from build123d import *
from OCP.BRepFilletAPI import BRepFilletAPI_MakeChamfer

# Parameters (mm, degrees)
SKETCH1_W           = 53
SKETCH1_H           = 5
SKETCH1_H_2         = 70
SKETCH1_R           = 1.5
BOSS_EXTRUDE1_DEPTH = 5
SKETCH2_R           = 1.5
CUT_EXTRUDE1_DEPTH  = 10
SKETCH3_R           = 3.5
CUT_EXTRUDE2_DEPTH  = 3
SKETCH2_3_W         = 2.25
SKETCH2_3_H         = 15
BOSS_EXTRUDE2_DEPTH = 6
CUT_EXTRUDE3_DEPTH  = 79.961729873
CHAMFER2_SIZE       = 0.75
CHAMFER2_SIZE_2     = 4.253461365
CHAMFER3_SIZE       = 1.1
CHAMFER3_SIZE_2     = 6.238410002
SKETCH5_W           = 15
SKETCH5_H           = 30
CUT_EXTRUDE4_DEPTH  = 3
FILLET1_R           = 10
CHAMFER4_SIZE       = 5


# Some blends are built 0.0001 mm under size
with BuildPart() as part:
    # Sketch1 → Boss-Extrude1 (new body)
    # profile 1 of 2: a face of its own
    with BuildSketch(Plane(origin=(0, 0, 0), x_dir=(1, 0, 0), z_dir=(0, 1, 0))):
        with Locations((5.35835502, -40.562169312)):
            Rectangle(SKETCH1_W, SKETCH1_H)
    # profile 2 of 2: a face of its own
    with BuildSketch(Plane(origin=(0, 0, 0), x_dir=(1, 0, 0), z_dir=(0, 1, 0))):
        with Locations((5.35835502, -3.062169312)):
            Rectangle(SKETCH1_W, SKETCH1_H_2)
        with Locations(Location((29.35835502, -24.362169312, 0), (0, 0, 270))):
            Circle(SKETCH1_R, mode=Mode.SUBTRACT)
        with Locations(Location((24.85835502, 27.437830688, 0), (0, 0, 270))):
            Circle(SKETCH1_R, mode=Mode.SUBTRACT)
        with Locations(Location((-3.14164498, 27.437830688, 0), (0, 0, 270))):
            Circle(SKETCH1_R, mode=Mode.SUBTRACT)
        with Locations(Location((-18.64164498, -23.062169312, 0), (0, 0, 270))):
            Circle(SKETCH1_R, mode=Mode.SUBTRACT)
    extrude(amount=BOSS_EXTRUDE1_DEPTH)

    # Sketch2 → Cut-Extrude1 (cut)
    with BuildSketch(Plane.XZ):
        with Locations(Location((5.35835502, 15.062169312, 0), (0, 0, 270))):
            Circle(SKETCH2_R)
    extrude(amount=-CUT_EXTRUDE1_DEPTH, mode=Mode.SUBTRACT)

    # Sketch3 → Cut-Extrude2 (cut)
    with BuildSketch(Plane(origin=(0, 5, 0), x_dir=(1, 0, 0), z_dir=(0, 1, 0))):
        with Locations(Location((5.35835502, -15.062169312, 0), (0, 0, 270))):
            Circle(SKETCH3_R)
    extrude(amount=-CUT_EXTRUDE2_DEPTH, mode=Mode.SUBTRACT)

    # Sketch2<3> → Boss-Extrude2 (add)
    with BuildSketch(Plane.XZ):
        with Locations((3.48335502, -2.437830688)):
            Rectangle(SKETCH2_3_W, SKETCH2_3_H)
        with Locations((7.23335502, -2.437830688)):
            Rectangle(SKETCH2_3_W, SKETCH2_3_H)
        with Locations((7.23335502, 32.562169312)):
            Rectangle(SKETCH2_3_W, SKETCH2_3_H)
        with Locations((3.48335502, 32.562169312)):
            Rectangle(SKETCH2_3_W, SKETCH2_3_H)
    extrude(amount=BOSS_EXTRUDE2_DEPTH)

    # Sketch4 → Cut-Extrude3 (cut, through all)
    with BuildSketch(Plane.XY.offset(40.062169312)):
        Polygon((8.35835502, -4.5), (8.35835502, 0), (7.65835502, 0), (7.65835502, -4), (8.05835502, -4.285714286), (8.05835502, -5.1), (7.15835502, -6), (8.35835502, -6), (8.35835502, -4.8), align=None)
        Polygon((2.65835502, -4.285714286), (3.05835502, -4), (3.05835502, 0), (2.35835502, 0), (2.35835502, -4.5), (2.35835502, -4.8), (2.35835502, -6), (3.55835502, -6), (2.65835502, -5.1), align=None)
    extrude(amount=-CUT_EXTRUDE3_DEPTH, mode=Mode.SUBTRACT)

    # Chamfer2
    chamfer2_edges_1 = [part.edges().sort_by_distance(p)[0] for p in [
        (4.60835502, 0, -2.437830688),
    ]]
    chamfer2_side_1 = [part.faces().sort_by_distance(p)[0] for p in [
        (4.62335502, 0, -2.437830688),
    ]]
    chamfer2_edges_2 = [part.edges().sort_by_distance(p)[0] for p in [
        (6.10835502, 0, -2.437830688),
    ]]
    chamfer2_side_2 = [part.faces().sort_by_distance(p)[0] for p in [
        (6.09335502, 0, -2.437830688),
    ]]
    chamfer2_edges_3 = [part.edges().sort_by_distance(p)[0] for p in [
        (6.10835502, 0, 32.562169312),
    ]]
    chamfer2_side_3 = [part.faces().sort_by_distance(p)[0] for p in [
        (6.09335502, 0, 32.562169312),
    ]]
    chamfer2_edges_4 = [part.edges().sort_by_distance(p)[0] for p in [
        (4.60835502, 0, 32.562169312),
    ]]
    chamfer2_side_4 = [part.faces().sort_by_distance(p)[0] for p in [
        (4.62335502, 0, 32.562169312),
    ]]
    chamfer2 = BRepFilletAPI_MakeChamfer(part.part.solid().wrapped)
    for e in chamfer2_edges_1:
        chamfer2.Add(CHAMFER2_SIZE - 0.0001, CHAMFER2_SIZE_2 - 0.0001, e.wrapped, chamfer2_side_1[0].wrapped)
    for e in chamfer2_edges_2:
        chamfer2.Add(CHAMFER2_SIZE - 0.0001, CHAMFER2_SIZE_2 - 0.0001, e.wrapped, chamfer2_side_2[0].wrapped)
    for e in chamfer2_edges_3:
        chamfer2.Add(CHAMFER2_SIZE - 0.0001, CHAMFER2_SIZE_2 - 0.0001, e.wrapped, chamfer2_side_3[0].wrapped)
    for e in chamfer2_edges_4:
        chamfer2.Add(CHAMFER2_SIZE - 0.0001, CHAMFER2_SIZE_2 - 0.0001, e.wrapped, chamfer2_side_4[0].wrapped)
    add(Compound.cast(chamfer2.Shape()), mode=Mode.REPLACE)  # a hair under: the kernel refuses the full size

    # Chamfer3
    # the kernel refuses this chamfer: 6.238410002, 1.1 mm, written as the material it takes off along each edge
    with BuildSketch(Plane(origin=(20.819105437, -6, 40.062169312), x_dir=(0, -0.210138760767435, -0.977671571246258), z_dir=(-1, 0, 0))) as chamfer3_piece_1_section:
        Polygon((CHAMFER3_SIZE * 0.977671571246, -CHAMFER3_SIZE * 0.210138760767), (-CHAMFER3_SIZE_2 * 0.210138760753, -CHAMFER3_SIZE_2 * 0.97767157118), (0, 0), align=None)
    chamfer3_piece_1 = extrude(amount=33.471500834, mode=Mode.PRIVATE)
    chamfer3_piece_1 = split(chamfer3_piece_1, bisect_by=Plane(origin=(4.08335502, 0, 39.758425896), z_dir=(0, -1, 0)), keep=Keep.TOP, mode=Mode.PRIVATE)
    add(chamfer3_piece_1, mode=Mode.SUBTRACT)
    with BuildSketch(Plane(origin=(-12.652395397, -6, 25.062169312), x_dir=(0, -0.210138760767435, 0.977671571246258), z_dir=(1, 0, 0))) as chamfer3_piece_2_section:
        Polygon((CHAMFER3_SIZE * 0.977671571246, -CHAMFER3_SIZE * 0.210138760767), (-CHAMFER3_SIZE_2 * 0.210138760753, -CHAMFER3_SIZE_2 * 0.97767157118), (0, 0), align=None)
    chamfer3_piece_2 = extrude(amount=33.471500834, mode=Mode.PRIVATE)
    chamfer3_piece_2 = split(chamfer3_piece_2, bisect_by=Plane(origin=(4.08335502, 0, 25.365912729), z_dir=(0, -1, 0)), keep=Keep.TOP, mode=Mode.PRIVATE)
    add(chamfer3_piece_2, mode=Mode.SUBTRACT)
    with BuildSketch(Plane(origin=(23.369105437, -6, 40.062169312), x_dir=(0, -0.210138760767435, -0.977671571246258), z_dir=(-1, 0, 0))) as chamfer3_piece_3_section:
        Polygon((CHAMFER3_SIZE * 0.977671571246, -CHAMFER3_SIZE * 0.210138760767), (-CHAMFER3_SIZE_2 * 0.210138760753, -CHAMFER3_SIZE_2 * 0.97767157118), (0, 0), align=None)
    chamfer3_piece_3 = extrude(amount=33.471500834, mode=Mode.PRIVATE)
    chamfer3_piece_3 = split(chamfer3_piece_3, bisect_by=Plane(origin=(6.63335502, 0, 39.758425896), z_dir=(0, -1, 0)), keep=Keep.TOP, mode=Mode.PRIVATE)
    add(chamfer3_piece_3, mode=Mode.SUBTRACT)
    with BuildSketch(Plane(origin=(-10.102395397, -6, 25.062169312), x_dir=(0, -0.210138760767435, 0.977671571246258), z_dir=(1, 0, 0))) as chamfer3_piece_4_section:
        Polygon((CHAMFER3_SIZE * 0.977671571246, -CHAMFER3_SIZE * 0.210138760767), (-CHAMFER3_SIZE_2 * 0.210138760753, -CHAMFER3_SIZE_2 * 0.97767157118), (0, 0), align=None)
    chamfer3_piece_4 = extrude(amount=33.471500834, mode=Mode.PRIVATE)
    chamfer3_piece_4 = split(chamfer3_piece_4, bisect_by=Plane(origin=(6.63335502, 0, 25.365912729), z_dir=(0, -1, 0)), keep=Keep.TOP, mode=Mode.PRIVATE)
    add(chamfer3_piece_4, mode=Mode.SUBTRACT)
    with BuildSketch(Plane(origin=(23.369105437, -6, 5.062169312), x_dir=(0, -0.21013876076743537, -0.9776715712462578), z_dir=(-1, 0, 0))) as chamfer3_piece_5_section:
        Polygon((CHAMFER3_SIZE * 0.977671571246, -CHAMFER3_SIZE * 0.210138760767), (-CHAMFER3_SIZE_2 * 0.210138760753, -CHAMFER3_SIZE_2 * 0.97767157118), (0, 0), align=None)
    chamfer3_piece_5 = extrude(amount=33.471500834, mode=Mode.PRIVATE)
    chamfer3_piece_5 = split(chamfer3_piece_5, bisect_by=Plane(origin=(6.63335502, 0, 4.758425896), z_dir=(0, -1, 0)), keep=Keep.TOP, mode=Mode.PRIVATE)
    add(chamfer3_piece_5, mode=Mode.SUBTRACT)
    with BuildSketch(Plane(origin=(-10.102395397, -6, -9.937830688), x_dir=(0, -0.21013876076743562, 0.9776715712462578), z_dir=(1, 0, 0))) as chamfer3_piece_6_section:
        Polygon((CHAMFER3_SIZE * 0.977671571246, -CHAMFER3_SIZE * 0.210138760767), (-CHAMFER3_SIZE_2 * 0.210138760753, -CHAMFER3_SIZE_2 * 0.97767157118), (0, 0), align=None)
    chamfer3_piece_6 = extrude(amount=33.471500834, mode=Mode.PRIVATE)
    chamfer3_piece_6 = split(chamfer3_piece_6, bisect_by=Plane(origin=(6.63335502, 0, -9.634087271), z_dir=(0, -1, 0)), keep=Keep.TOP, mode=Mode.PRIVATE)
    add(chamfer3_piece_6, mode=Mode.SUBTRACT)
    with BuildSketch(Plane(origin=(20.819105437, -6, 5.062169312), x_dir=(0, -0.21013876076743546, -0.9776715712462578), z_dir=(-1, 0, 0))) as chamfer3_piece_7_section:
        Polygon((CHAMFER3_SIZE * 0.977671571246, -CHAMFER3_SIZE * 0.210138760767), (-CHAMFER3_SIZE_2 * 0.210138760753, -CHAMFER3_SIZE_2 * 0.97767157118), (0, 0), align=None)
    chamfer3_piece_7 = extrude(amount=33.471500834, mode=Mode.PRIVATE)
    chamfer3_piece_7 = split(chamfer3_piece_7, bisect_by=Plane(origin=(4.08335502, 0, 4.758425896), z_dir=(0, -1, 0)), keep=Keep.TOP, mode=Mode.PRIVATE)
    add(chamfer3_piece_7, mode=Mode.SUBTRACT)
    with BuildSketch(Plane(origin=(-12.652395397, -6, -9.937830688), x_dir=(-1.5437276286848704e-15, -0.21013876076743562, 0.9776715712462578), z_dir=(1, 0, 0))) as chamfer3_piece_8_section:
        Polygon((CHAMFER3_SIZE * 0.977671571246, -CHAMFER3_SIZE * 0.210138760767), (-CHAMFER3_SIZE_2 * 0.210138760753, -CHAMFER3_SIZE_2 * 0.97767157118), (0, 0), align=None)
    chamfer3_piece_8 = extrude(amount=33.471500834, mode=Mode.PRIVATE)
    chamfer3_piece_8 = split(chamfer3_piece_8, bisect_by=Plane(origin=(4.08335502, 0, -9.634087271), z_dir=(0, -1, 0)), keep=Keep.TOP, mode=Mode.PRIVATE)
    add(chamfer3_piece_8, mode=Mode.SUBTRACT)

    # Sketch5 → Cut-Extrude4 (cut)
    with BuildSketch(Plane.XZ):
        with Locations((24.35835502, 5.062169312)):
            Rectangle(SKETCH5_W, SKETCH5_H)
        with Locations((-13.64164498, 5.062169312)):
            Rectangle(SKETCH5_W, SKETCH5_H)
    extrude(amount=-CUT_EXTRUDE4_DEPTH, mode=Mode.SUBTRACT)

    # Fillet1
    # the kernel refuses this fillet: 10 mm, written as the material it adds along each edge
    with BuildSketch(Plane(origin=(31.85835502, 3, -9.937830688), x_dir=(0, -1, 0), z_dir=(-1, 0, 0))) as fillet1_piece_1:
        with BuildLine():
            CenterArc((10, 7.141428429), FILLET1_R, 180, 45.572995999)
            Line((0, 7.141428429), (0, 0))
            Line((0, 0), (3, 0))
        make_face()
    extrude(amount=32.853571071)
    with BuildSketch(Plane(origin=(16.85835502, 3, 20.062169312), x_dir=(0, -1, 0), z_dir=(1, 0, 0))) as fillet1_piece_2:
        with BuildLine():
            CenterArc((10, 7.141428429), FILLET1_R, 180, 45.572995999)
            Line((0, 7.141428429), (0, 0))
            Line((0, 0), (3, 0))
        make_face()
    extrude(amount=15)
    with BuildSketch(Plane(origin=(-6.14164498, 3, 20.062169312), x_dir=(0, -1, 0), z_dir=(-1, 0, 0))) as fillet1_piece_3:
        with BuildLine():
            CenterArc((10, -7.141428429), FILLET1_R, 134.427004001, 45.572995999)
            Line((0, -7.141428429), (0, 0))
            Line((0, 0), (3, 0))
        make_face()
    extrude(amount=15)
    with BuildSketch(Plane(origin=(-21.14164498, 3, -9.937830688), x_dir=(0, -1, 0), z_dir=(1, 0, 0))) as fillet1_piece_4:
        with BuildLine():
            CenterArc((10, -7.141428429), FILLET1_R, 134.427004001, 45.572995999)
            Line((0, -7.141428429), (0, 0))
            Line((0, 0), (3, 0))
        make_face()
    extrude(amount=32.853571071)
    with BuildSketch(Plane(origin=(-6.14164498, 3, -27.791401759), x_dir=(0, -1, 0), z_dir=(0, 0, 1))) as fillet1_piece_5:
        with BuildLine():
            CenterArc((10, -7.141428429), FILLET1_R, 134.427004001, 45.572995999)
            Line((0, -7.141428429), (0, 0))
            Line((0, 0), (3, 0))
        make_face()
    extrude(amount=65.707142143)
    with BuildSketch(Plane(origin=(16.85835502, 3, -9.937830688), x_dir=(0, -1, 0), z_dir=(0, 0, 1))) as fillet1_piece_6:
        with BuildLine():
            CenterArc((10, 7.141428429), FILLET1_R, 180, 45.572995999)
            Line((0, 7.141428429), (0, 0))
            Line((0, 0), (3, 0))
        make_face()
    extrude(amount=47.853571071)

    # Chamfer4
    chamfer4_edges = [part.edges().sort_by_distance(p)[0] for p in [
        (31.85835502, 2.5, 43.062169312),
        (-21.14164498, 2.5, 43.062169312),
        (-21.14164498, 2.5, -31.937830688),
        (31.85835502, 2.5, -31.937830688),
    ]]
    chamfer(chamfer4_edges, length=CHAMFER4_SIZE)


solid = part.part
Can you work these out from the model? Positions are in its coordinate system, mm. A direction names the side the tool comes from. Coordinates: 2 decimals unless noted, no trailing zeros. Order: outer loops, then holes, each group sorted by start corner. A loop starts at its lowest first (then second) coordinate and runs counter-clockwise, first axis right, second up. Notation, with made-up numbers: (-22, 65) -> (29, 65) arc R7 ccw to (29, 69) -> close; hole circle Ø2 at (67, -7). An arc over 180 degrees is marked (long way). Use one line per item in the form item = value.
Q1. I need wall thicknesses on L1, parallel to Y at x = -6, z = 17; L2, parallel to X at y = -4.75, z = 39; L3, parallel to X at y = -1, z = 30.5. Which ranges of each line are inside material? Lowest first, please.
From the geometry:
L1 = 0 to 5
L2 = 2.66 to 4.61, 6.11 to 8.06
L3 = 3.06 to 5.18, 5.53 to 7.66
Q2. Imagine slicing it at A-A, the plane y = -1.5. List the corners of the cut face in (x, z) for me, then the cut area to 3 significant figures.
From the geometry:
outline = (3.06, -9.63) -> (5.09, -9.63) -> (5.09, 4.76) -> (3.06, 4.76) -> close; (3.06, 25.37) -> (5.09, 25.37) -> (5.09, 39.76) -> (3.06, 39.76) -> close; (5.62, -9.63) -> (7.66, -9.63) -> (7.66, 4.76) -> (5.62, 4.76) -> close; (5.62, 25.37) -> (7.66, 25.37) -> (7.66, 39.76) -> (5.62, 39.76) -> close
area = 117 mm²
Q3. Imagine slicing it at C-C, the plane x = 15.5. List the corners of the cut face in (y, z) for me.
From the geometry:
outline = (0, -31.94) -> (5, -31.94) -> (5, 43.06) -> (0, 43.06) -> close
Q4. Which directions (+Z, -Z, +X, -X, +Y, -Y) give clear straight access to the entire face, cutting with the end or side of a thin tool? Please do faces 1 (the face through (7.658, -2, 33)), 2 (the face through (6.108, -5, -3)), 3 (the face through (-15.41, 2.2, -6.72)).
From the geometry:
face_1 = +Z, -Z, +X
face_2 = +Z, -Z, -Y
face_3 = -X, -Y
Q5. Imagine slicing it at D-D, the plane z = 7.5. List the corners of the cut face in (x, y) for me, then the cut area to 3 significant figures.
From the geometry:
outline = (-21.14, 3) -> (-13.28, 3) arc R10 cw to (-6.14, 0) -> (16.86, 0) arc R10 cw to (24, 3) -> (31.86, 3) -> (31.86, 5) -> (-21.14, 5) -> close
area = 188 mm²
Q6. We'd pull the mould along Z, two halves only. Please class faces 4 (the face through (-4.606, 2.465, -27.763)), 5 (the face through (5, 2, 17)), 6 (the face through (-18.607, 2.465, 40.597)), 7 (the face through (-21.142, 4, 5)): released by +Z, released by -Z, zero draft, split by the parting line, or undercut.
From the geometry:
face_4 = undercut
face_5 = undercut
face_6 = released by +Z
face_7 = zero draft
Q7. Will these pins go through, and if not, where does the flat tip stop? P1, Ø4, axis at y = 1.5, z = 10.5, coming from the +X side; P2, Ø4, axis at x = 5.36, z = 15.06, coming from the -Y side; P3, Ø0.5, axis at y = -5, z = 0.5, coming from the -X side; P4, Ø6.5, axis at x = -15.5, z = 8.5, coming from the -Y side.
From the geometry:
P1 = 31.86
P2 = 0
P3 = 2.66
P4 = 2.95
